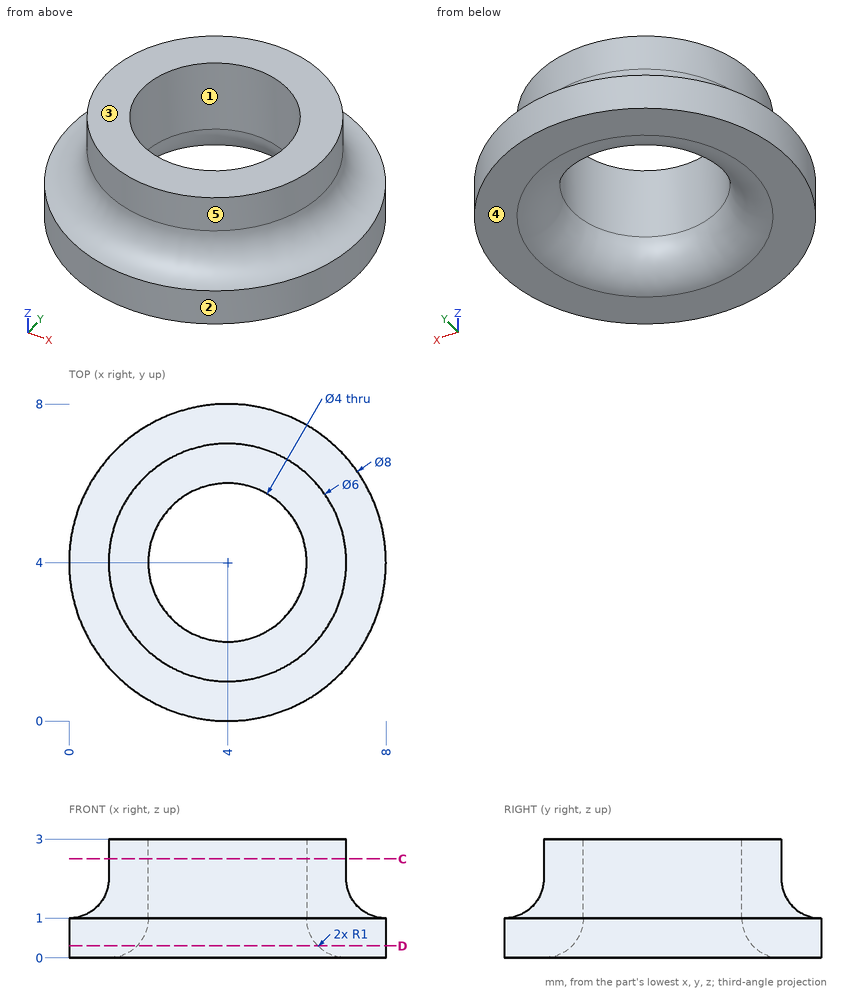
The drawing under review shows one solid part. Ordinate dimensions are in mm from its lowest x, y, z. A direction names the side the tool comes from. Coordinates: 2 decimals unless noted, no trailing zeros. Order: outer loops, then holes, each group sorted by start corner. A loop starts at its lowest first (then second) coordinate and runs counter-clockwise, first axis right, second up. Notation, with made-up numbers: (-15, -37.75) -> (-1, -37.75) arc R12 cw to (-1, -16.75) -> close; hole circle Ø2 at (-7, -7). An arc over 180 degrees is marked (long way). Return JSON: item names as keys, results as strings.
1. For line 1 (Y direction, x = 4, z = 2.6); line 2 (Y direction, x = 4, z = 1.2); line 3 (X direction, y = 5.25, z = 2.25), list the stretches that pass through material, from the lowest coordinate up. Write a range as from..to.
Answer block:
{"line 1": "1..2, 6..7", "line 2": "0.6..2, 6..7.4", "line 3": "1.27..2.44, 5.56..6.73"}
2. Machinability: for the marked faces 4 and 5, which of the approach directions +Z, -Z, +X, -X, +Y, -Y give a long, thin tool a straight path to every point of the face, cutting with its end or side? Answer none if there is none.
Answer block:
{"face 4": "-Z, +X, -X, +Y, -Y", "face 5": "+Z"}
3. For pin 1 Ø1 at (x, y) = (4, 6) entering from -Z; pin 2 Ø1.5 at (x, z) = (1.5, 2) entering from +Y, all flat-tipped, find the tip position at first contact; note any pin that passes through.
Answer block:
{"pin 1": "z = 0.13", "pin 2": "y = 6.46"}
4. We need section D-D on z = 0.3. Write out the cut boundary in (x, y).
Answer block:
{"outline": "circle Ø8 at (4, 4); hole circle Ø4.57 at (4, 4)"}
5. The part is to be moulded in two halves that separate along X. For the marked faces 1, 2 and 3, say which applies: +X half, -X half, draft (parallel to the pull), parting line (faces both ways), or undercut.
Answer block:
{"face 1": "undercut", "face 2": "parting line", "face 3": "draft"}
6. We need section C-C on z = 2.5. Write out the cut boundary in (x, y), and give its area (3 significant figures).
Answer block:
{"outline": "circle Ø6 at (4, 4); hole circle Ø4 at (4, 4)", "area": "15.7 mm²"}
